```python
from build123d import *

# Parameters (mm, degrees)
BOX008_W          = 58
BOX008_H          = 10
BOX008_DEPTH      = 3
CONE_PITCH_ANGLE  = 90
CYLINDER001_R     = 6
CYLINDER001_DEPTH = 4
CYLINDER_R        = 8
CYLINDER_DEPTH    = 4
PAD001_DEPTH      = 15
SKETCH_R          = 12
SKETCH_R_2        = 1.6
PAD_DEPTH         = 20
CHAMFER003_SIZE   = 2
FILLET_R          = 5


with BuildPart() as obj1:
    # Box008 → Box008 (new body)
    with BuildSketch(Plane(origin=(3, 0, 3), x_dir=(1, 0, 0), z_dir=(0, 0, 1))):
        with Locations((29, 5)):
            Rectangle(BOX008_W, BOX008_H)
    extrude(amount=BOX008_DEPTH)


with BuildPart() as cone_forat_cargol003:
    # Cone002 → Cone002 (revolve)
    with BuildSketch(Plane(origin=(55, 5, 0), x_dir=(1, 0, 0), z_dir=(0, -1, 0))):
        Polygon((0, 0), (3, 0), (1.75, 3), (0, 3), align=None)
    revolve(axis=Axis((55, 5, 0), (0, 0, 1)))


with BuildPart() as cone_forat_cargol002:
    # Cone001 → Cone001 (revolve)
    with BuildSketch(Plane(origin=(25, 5, 0), x_dir=(1, 0, 0), z_dir=(0, -1, 0))):
        Polygon((0, 0), (3, 0), (1.75, 3), (0, 3), align=None)
    revolve(axis=Axis((25, 5, 0), (0, 0, 1)))


with BuildPart() as cone_forat_cargol001:
    # Cone → Cone (revolve)
    with BuildSketch(Plane.XZ):
        Polygon((0, 0), (3, 0), (1.75, 3), (0, 3), align=None)
    revolve(axis=Axis((0, 0, 0), (0, 0, 1)))


with BuildPart() as cone_forat_cargol001_1:
    # Cone pitch: moved
    add(cone_forat_cargol001.part.rotate(Axis((0, 0, 0), (0, 1, 0)), CONE_PITCH_ANGLE))


with BuildPart() as cone_forat_cargol001_2:
    # Cone placement: moved
    add(cone_forat_cargol001_1.part.moved(Location((0, 5, 10))))


with BuildPart() as cyl_brida_int:
    # Cylinder001 → Cylinder001 (new body)
    with BuildSketch(Plane.XY):
        Circle(CYLINDER001_R)
    extrude(amount=CYLINDER001_DEPTH)


with BuildPart() as cyl_brida_ext:
    # Cylinder → Cylinder (new body)
    with BuildSketch(Plane.XY):
        Circle(CYLINDER_R)
    extrude(amount=CYLINDER_DEPTH)


with BuildPart() as obj2:
    # Cut002 base: copy of Cyl-brida-ext
    add(cyl_brida_ext.part)

    # Cut002: cut Cyl-brida-int
    add(cyl_brida_int.part, mode=Mode.SUBTRACT)


with BuildPart() as obj2_1:
    # Cut002 placement: moved
    add(obj2.part.moved(Location((10, 30, 12))))


with BuildPart() as obj3:
    # Cut001 base: copy of Cyl-brida-ext
    add(cyl_brida_ext.part)

    # Cut001: cut Cyl-brida-int
    add(cyl_brida_int.part, mode=Mode.SUBTRACT)


with BuildPart() as obj3_1:
    # Cut001 placement: moved
    add(obj3.part.moved(Location((10, 30, 4))))


with BuildPart() as obj4:
    # Sketch001 → Pad001 (new body)
    with BuildSketch(Plane.XY.offset(5)):
        Polygon((3, 10), (21, 10), (21, 50), (61, 50), (61, 0), (3, 0), align=None)
    extrude(amount=PAD001_DEPTH)


with BuildPart() as y_end_motor:
    # Sketch → Pad (new body)
    with BuildSketch(Plane.XY):
        with BuildLine():
            ThreePointArc((6.75, 30), (11, 25.75), (15.25, 30))
            Line((15.25, 30), (21, 30))
            Line((21, 30), (21, 50))
            Line((21, 50), (61, 50))
            Line((61, 50), (61, 0))
            Line((0, 0), (61, 0))
            Line((0, 30), (0, 0))
            Line((6.75, 30), (0, 30))
        make_face()
        with Locations((41, 30)):
            Circle(SKETCH_R, mode=Mode.SUBTRACT)
        with Locations((25.500268, 45.500268)):
            Circle(SKETCH_R_2, mode=Mode.SUBTRACT)
        with Locations((25.499732, 14.500268)):
            Circle(SKETCH_R_2, mode=Mode.SUBTRACT)
        with Locations((56.499732, 14.499732)):
            Circle(SKETCH_R_2, mode=Mode.SUBTRACT)
        with Locations((56.500268, 45.499732)):
            Circle(SKETCH_R_2, mode=Mode.SUBTRACT)
    extrude(amount=PAD_DEPTH)

    # Cut: cut obj4
    add(obj4.part, mode=Mode.SUBTRACT)

    # Cut003: cut obj3
    add(obj3_1.part, mode=Mode.SUBTRACT)

    # Cut004: cut obj2
    add(obj2_1.part, mode=Mode.SUBTRACT)

    # Cut005: cut Cone-forat-cargol001
    add(cone_forat_cargol001_2.part, mode=Mode.SUBTRACT)

    # Cut006: cut Cone-forat-cargol002
    add(cone_forat_cargol002.part, mode=Mode.SUBTRACT)

    # Cut007: cut Cone-forat-cargol003
    add(cone_forat_cargol003.part, mode=Mode.SUBTRACT)

    # Cut027: cut obj1
    add(obj1.part, mode=Mode.SUBTRACT)

    # Chamfer003
    chamfer003_edges = [y_end_motor.edges().sort_by_distance(p)[0] for p in [
        (21, 20, 5),
    ]]
    chamfer(chamfer003_edges, length=CHAMFER003_SIZE)

    # Fillet
    fillet_edges = [y_end_motor.edges().sort_by_distance(p)[0] for p in [
        (21, 50, 2.5),
        (61, 50, 2.5),
    ]]
    fillet(fillet_edges, radius=FILLET_R)


with BuildPart() as part_mirroring:
    # Part__Mirroring: instance of y-end-motor
    add(y_end_motor.part.mirror(Plane(origin=(0, 0, 0), x_dir=(0, -1, 0), z_dir=(1, 0, 0))))


solid = part_mirroring.part
```
Design review of the part built by this model. Coordinates are the model's own, in mm. A direction names the side the tool comes from. Round coordinates to 2 decimals unless told otherwise and drop trailing zeros. Write each loop counter-clockwise with the first axis right and the second up, starting at its lowest first coordinate (ties: lowest second). Pieces come first, ordered by that corner, then holes. Notation, with made-up numbers: (2, 2.25) -> (37, 2.25) arc R27 cw to (37, 41.25) -> close; hole circle Ø7 at (-37, -18). An arc over 180 degrees is marked (long way). Answer in a Markdown table with one row per item.
Q1. Take a section at D-D, the plane x = -25. State the section outline as (y, z) points, then the cut area to 3 significant figures.
The answers:
| item | result |
|---|---|
| outline | (0, 0) -> (2, 0) -> (3.25, 3) -> (0, 3) -> close; (6.75, 3) -> (8, 0) -> (12.98, 0) -> (12.98, 5) -> (10, 5) -> (10, 3) -> close; (16.02, 0) -> (43.98, 0) -> (43.98, 5) -> (16.02, 5) -> close; (47.02, 0) -> (49.9, 0) -> (49.9, 5) -> (47.02, 5) -> close |
| area | 185 mm² |
Q2. To check wall thickness, follow L1, parallel to Z at x = -16.5, y = 28; L2, parallel to Y at x = -41, z = 1.5; L3, parallel to Y at x = -41, z = 3.65. State the ranges of each line that lie inside material, in increasing order. Write a range as [from, to].
The answers:
| item | result |
|---|---|
| L1 | [0, 4], [8, 12], [16, 20] |
| L2 | [0, 18], [42, 50] |
| L3 | [10, 18], [42, 50] |
Q3. Take a section at B-B, the plane x = -41. State the section outline as (y, z) points, then the cut area to 3 significant figures.
The answers:
| item | result |
|---|---|
| outline | (0, 0) -> (18, 0) -> (18, 5) -> (10, 5) -> (10, 3) -> (0, 3) -> close; (42, 0) -> (50, 0) -> (50, 5) -> (42, 5) -> close |
| area | 110 mm² |
Q4. For faces 1 (the face through (-8.8, 23.9, 8)), 2 (the face through (-52.085, 25.404, 2.465)), 3 (the face through (-3, 5, 13)), 4 (the face through (-3, 30, 10)), 5 (the face through (-21, 20, 13)), list the 3-axis set-ups (+Z, -Z, +X, -X, +Y, -Y) from which the entire face can be reached by the end or side of a thin tool; tool diameter is ignored.
The answers:
| item | result |
|---|---|
| face 1 | none |
| face 2 | +Z, -Z |
| face 3 | +Z, -X, -Y |
| face 4 | +Z, -Z, +X, +Y |
| face 5 | +Z, -X, +Y, -Y |
Q5. Take a section at C-C, the plane z = 10. State the section outline as (x, y) points.
The answers:
| item | result |
|---|---|
| outline | (-21, 10) -> (-3, 10) -> (-3, 6.75) -> (0, 8) -> (0, 30) -> (-6.75, 30) arc R4.25 cw to (-15.25, 30) -> (-21, 30) -> close; (-3, 0) -> (0, 0) -> (0, 2) -> (-3, 3.25) -> close |
Q6. Clearance check with flat-ended pins moving along their axes: pin 1 Ø1.9 at (x, y) = (-56.5, 14.5) entering from -Z; pin 2 Ø5 at (x, y) = (-56.5, 45.5) entering from +Z; pin 3 Ø6 at (y, z) = (30.5, 14.5) entering from -X; pin 4 Ø1.5 at (y, z) = (40.5, 1.5) entering from +X. State where each tip first meets the part, or that it passes through.
The answers:
| item | result |
|---|---|
| pin 1 | through |
| pin 2 | z = 5 |
| pin 3 | x = -21 |
| pin 4 | x = -21 |
Q7. Draft analysis for pull direction X (two halves, no side actions). For faces 6 (the face through (-22, 20, 6)), 7 (the face through (-10, 24, 14)), 8 (the face through (-11, 19, 20)), state which applies: +X half, -X half, draft (parallel to the pull), parting line (faces both ways), or undercut.
The answers:
| item | result |
|---|---|
| face 6 | -X half |
| face 7 | undercut |
| face 8 | draft |
Q8. Take a section at A-A, the plane y = 28.5. Count the separate pieces of the cut face and the enclosed holes in it, then the cut area to 3 significant figures.
The answers:
| item | result |
|---|---|
| separate pieces | 3 |
| enclosed holes | 4 |
| area | 311 mm² |
